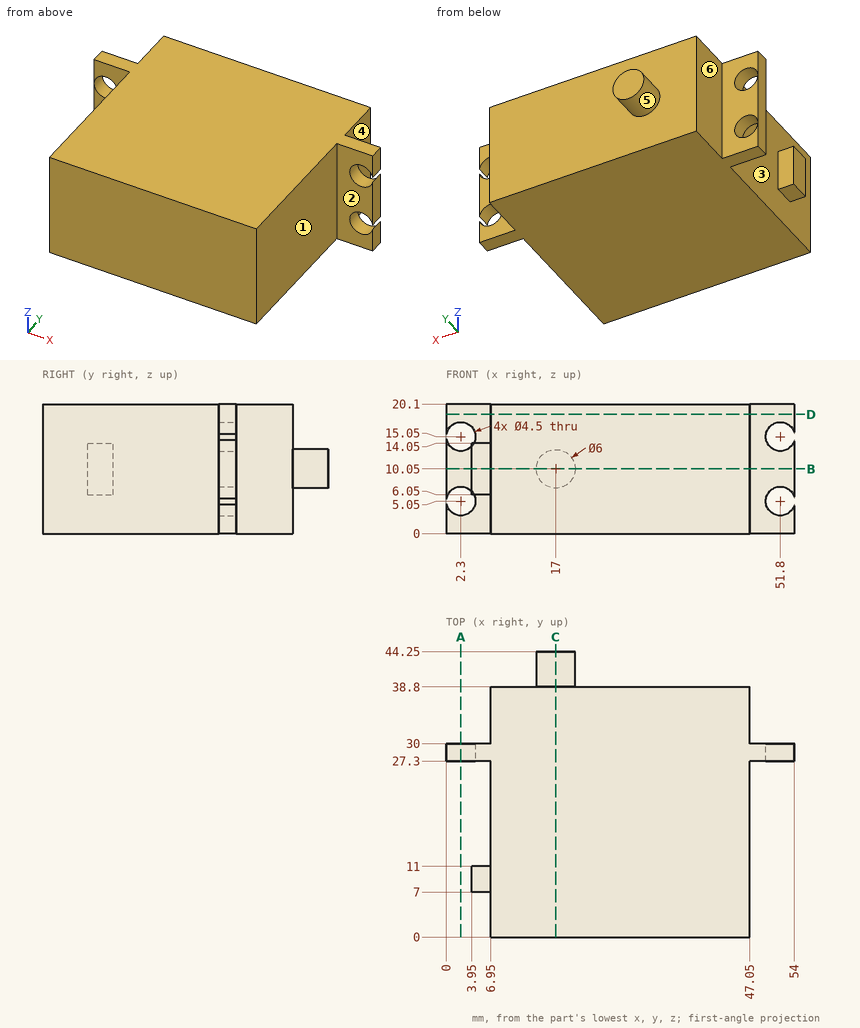
For this review, use the dimensioned drawing (mm, ordinates from the lowest corner) and the shaded views. A direction names the side the tool comes from. Coordinates: 2 decimals unless noted, no trailing zeros. Order: outer loops, then holes, each group sorted by start corner. A loop starts at its lowest first (then second) coordinate and runs counter-clockwise, first axis right, second up. Notation, with made-up numbers: (87, -22.5) - (91, -22.5) arc R29 ccw to (91, 7.5) - close; hole circle Ø4 at (26.25, -10). An arc over 180 degrees is marked (long way). Answer as a JSON object with one key per item and string values. Group by question number.
1. We need section A-A on x = 2.3. State the section outline as (y, z) points.
2. Clearance check with flat-ended pins moving along their axes: P1, Ø4.5, axis at y = 32.5, z = 10.5, coming from the -X side; P2, Ø0.9, axis at x = 5, y = 8, coming from the -Z side; P3, Ø1.2, axis at y = 9, z = 10.5, coming from the -X side. State where each tip first meets the part, or that it passes through.
3. We need section D-D on z = 18.5. State the section outline as (x, y) points.
4. We need section C-C on x = 17. State the section outline as (y, z) points, then the cut area to 3 significant figures.
5. The part is to be moulded in two halves that separate along Y. For the marked faces 1, 2 and 3, say which applies: pulls with the +Y half, pulls with the -Y half, needs draft (parallel to the pull), parting line crosses it, or undercut.
6. For probe 1 along Z at (x, y) = (2.3, 28.6); probe 2 along Y at (x, z) = (48.5, 17); probe 3 along Y at (x, z) = (38, 7.5), list the stretches that pass through material, from the lowest coordinate up.
7. For the marked faces 4, 5 and 6, list the 3-axis set-ups (+Z, -Z, +X, -X, +Y, -Y) from which the entire face can be reached by the end or side of a thin tool; tool diameter is ignored.
8. We need section B-B on z = 10.05. State the section outline as (x, y) points.
Final values:
{
 "1": {"outline": "(27.3, 0) - (30, 0) - (30, 2.8) - (27.3, 2.8) - close; (27.3, 7.3) - (30, 7.3) - (30, 12.8) - (27.3, 12.8) - close; (27.3, 17.3) - (30, 17.3) - (30, 20.1) - (27.3, 20.1) - close"},
 "2": {"P1": "x = 6.95", "P2": "z = 6.05", "P3": "x = 3.95"},
 "3": {"outline": "(0, 27.3) - (6.95, 27.3) - (6.95, 0) - (47.05, 0) - (47.05, 27.3) - (54, 27.3) - (54, 30) - (47.05, 30) - (47.05, 38.8) - (6.95, 38.8) - (6.95, 30) - (0, 30) - close"},
 "4": {"outline": "(0, 0) - (38.8, 0) - (38.8, 7.05) - (44.25, 7.05) - (44.25, 13.05) - (38.8, 13.05) - (38.8, 20.1) - (0, 20.1) - close", "area": "813 mm²"},
 "5": {"face 1": "needs draft", "face 2": "pulls with the -Y half", "face 3": "undercut"},
 "6": {"probe 1": "0 to 2.8, 7.3 to 12.8, 17.3 to 20.1", "probe 2": "27.3 to 30", "probe 3": "0 to 38.8"},
 "7": {"face 4": "+Z, -Z, +X, +Y", "face 5": "+Y", "face 6": "+Z, -Z, -X, +Y"},
 "8": {"outline": "(0, 27.3) - (6.95, 27.3) - (6.95, 11) - (3.95, 11) - (3.95, 7) - (6.95, 7) - (6.95, 0) - (47.05, 0) - (47.05, 27.3) - (54, 27.3) - (54, 30) - (47.05, 30) - (47.05, 38.8) - (20, 38.8) - (20, 44.25) - (14, 44.25) - (14, 38.8) - (6.95, 38.8) - (6.95, 30) - (0, 30) - close"}
}
